```python
from build123d import *

# Parameters (mm, degrees)
F0_R          = 80
F1_DEPTH      = 50
F2_R          = 4
F3_DEPTH      = 25
F4_SIZE       = 1
F5_W          = 3
F5_H          = 35
F6_DEPTH      = 100
F6_DEPTH_BACK = 100


with BuildPart() as f1:
    # F0 (on Top) → F1 (new body)
    with BuildSketch(Plane.XY):
        Circle(F0_R)
    extrude(amount=F1_DEPTH)

    # F2 (on Top) → F3 (cut)
    with BuildSketch(Plane.XY):
        with Locations((-49.497475, 49.497475)):
            Circle(F2_R)
        with Locations((-49.497475, -49.497475)):
            Circle(F2_R)
        with Locations((49.497475, 49.497475)):
            Circle(F2_R)
        with Locations((49.497475, -49.497475)):
            Circle(F2_R)
    extrude(amount=F3_DEPTH, mode=Mode.SUBTRACT)

    # F4
    f4_edges = [f1.edges().sort_by_distance(p)[0] for p in [
        (-80, 0, 50),
    ]]
    chamfer(f4_edges, length=F4_SIZE)

    # F5 (on Front) → F6 (cut, two sides)
    with BuildSketch(Plane.XZ) as f6_sk:
        with Locations((-63, 42.5)):
            Rectangle(F5_W, F5_H)
        with Locations((-57, 42.5)):
            Rectangle(F5_W, F5_H)
        with Locations((-51, 42.5)):
            Rectangle(F5_W, F5_H)
        with Locations((-45, 42.5)):
            Rectangle(F5_W, F5_H)
        with Locations((-39, 42.5)):
            Rectangle(F5_W, F5_H)
        with Locations((-33, 42.5)):
            Rectangle(F5_W, F5_H)
        with Locations((-27, 42.5)):
            Rectangle(F5_W, F5_H)
        with Locations((-21, 42.5)):
            Rectangle(F5_W, F5_H)
        with Locations((-15, 42.5)):
            Rectangle(F5_W, F5_H)
        with Locations((-9, 42.5)):
            Rectangle(F5_W, F5_H)
        with Locations((-3, 42.5)):
            Rectangle(F5_W, F5_H)
        with Locations((3, 42.5)):
            Rectangle(F5_W, F5_H)
        with Locations((9, 42.5)):
            Rectangle(F5_W, F5_H)
        with Locations((15, 42.5)):
            Rectangle(F5_W, F5_H)
        with Locations((21, 42.5)):
            Rectangle(F5_W, F5_H)
        with Locations((27, 42.5)):
            Rectangle(F5_W, F5_H)
        with Locations((33, 42.5)):
            Rectangle(F5_W, F5_H)
        with Locations((39, 42.5)):
            Rectangle(F5_W, F5_H)
        with Locations((45, 42.5)):
            Rectangle(F5_W, F5_H)
        with Locations((51, 42.5)):
            Rectangle(F5_W, F5_H)
        with Locations((57, 42.5)):
            Rectangle(F5_W, F5_H)
        with Locations((63, 42.5)):
            Rectangle(F5_W, F5_H)
    extrude(amount=F6_DEPTH, mode=Mode.SUBTRACT)
    extrude(f6_sk.sketch, amount=-F6_DEPTH_BACK, mode=Mode.SUBTRACT)


solid = f1.part
```
The model under review builds one solid part; all positions refer to its coordinate system, in mm. A direction names the side the tool comes from. Round coordinates to 2 decimals unless told otherwise and drop trailing zeros. Loops run counter-clockwise (first coordinate to the right, second up) from the corner with the lowest first, then second, coordinate; pieces in that order, holes last.
Item 1: For line 1 (Z direction, x = -51, y = -5); line 2 (Y direction, x = 54, z = 36.5); line 3 (Y direction, x = 69, z = 47.5), list the stretches that pass through material, from the lowest coordinate up.
Determined:
line 1: z = 0 to 25
line 2: y = -59.03 to 59.03
line 3: y = -40.48 to 40.48
Item 2: Take a section at B-B (z = 6). Write out the cut boundary in (x, y).
Determined:
outline: circle Ø160 at (0, 0); hole circle Ø8 at (-49.5, -49.5); hole circle Ø8 at (-49.5, 49.5); hole circle Ø8 at (49.5, -49.5); hole circle Ø8 at (49.5, 49.5)
Item 3: Mouldability with a two-part tool opening along X and no side actions: class faces 1 (the face through (-1, 1, 0)), 2 (the face through (-46.5, 1, 37)), 3 (the face through (73.9, -30.64, 24.16)) as released by +X, released by -X, zero draft, split by the parting line, or undercut.
Determined:
face 1: zero draft
face 2: undercut
face 3: split by the parting line
Item 4: Clearance check with flat-ended pins moving along their axes: pin 1 Ø1.5 at (x, y) = (45, -26.5) entering from +Z; pin 2 Ø3 at (y, z) = (-21.5, 38) entering from +X; pin 3 Ø7.5 at (y, z) = (7, 42) entering from +X. State where each tip first meets the part, or that it passes through.
Determined:
pin 1: stops at z = 25
pin 2: stops at x = 77.46
pin 3: stops at x = 79.93
Item 5: For faces 4 (the face through (49.5, 1, 37)), 5 (the face through (46.55, 52.2, 12.32)), 6 (the face through (-70, 1, 50)), list the 3-axis set-ups (+Z, -Z, +X, -X, +Y, -Y) from which the entire face can be reached by the end or side of a thin tool; tool diameter is ignored.
Determined:
face 4: +Z, +Y, -Y
face 5: -Z
face 6: +Z, +X, -X, +Y, -Y
Item 6: Take a section at A-A (z = 43.5). Give the number of separate pieces and of enclosed holes in the cut face, then the cut area to 3 significant figures.
Determined:
separate pieces: 23
enclosed holes: 0
area: 10,900 mm2
